For this review, take the finished solid that the model builds, in its own axes (mm). Face numbers are marked on the shaded views. A direction names the side the tool comes from. Coordinates: 2 decimals unless noted, no trailing zeros. Write each loop counter-clockwise with the first axis right and the second up, starting at its lowest first coordinate (ties: lowest second). Pieces come first, ordered by that corner, then holes. Notation, with made-up numbers: (80.5, 37) -> (117.5, 37) arc R23 cw to (117.5, 62) -> close; hole circle Ø3 at (80, 83.5). An arc over 180 degrees is marked (long way). Put each result on its own line as item: value. Start each with the question number.
Item 1: Consider section A-A on x = 0. Give the boundary of the cut face in (y, z).
Item 2: Insertion check: P1, Ø1, axis at y = 7, z = 1, coming from the -X side; P2, Ø1, axis at y = 0, z = 5, coming from the -X side; P3, Ø4, axis at x = 7, z = 1, coming from the +Y side; P4, Ø4, axis at y = -8.5, z = 1.5, coming from the -X side. Each pin has a flat end and moves straight along its axis. Give the tip position at first contact, or say it passes through.
Item 3: The part is to be moulded in two halves that separate along Y. For the marked faces 1, 2 and 3, say which applies: +Y half, -Y half, draft (parallel to the pull), parting line (faces both ways), or undercut.
Item 4: Consider section D-D on x = 3.25. Give the boundary of the cut face in (y, z), and give its area (3 significant figures).
Item 5: Consider section C-C on y = 0. Give the boundary of the cut face in (x, z), and give its area (3 significant figures).
Item 6: For the marked faces 4 and 5, list the 3-axis set-ups (+Z, -Z, +X, -X, +Y, -Y) from which the entire face can be reached by the end or side of a thin tool; tool diameter is ignored.
Item 7: To check wall thickness, follow L1, parallel to Y at x = 0, z = 4.5; L2, parallel to Z at x = 7, y = -9.5; L3, parallel to Y at x = 6.25, z = -2.5. State the ranges of each line that lie inside material, in increasing order.
Item 8: Consider section B-B on z = 7. Give the boundary of the cut face in (x, y).
```python
from build123d import *

# Parameters (mm, degrees)
SKETCH_2_R          = 4.5
EXTRUDE_1_DEPTH     = 9
SKETCH_3_R          = 15
EXTRUDE_2_DEPTH     = 3
CUT_EXTRUDE_1_DEPTH = 10


with BuildPart() as part:
    # Эскиз2 → Бобышка-Вытянуть1 (new body)
    with BuildSketch(Plane.XY):
        Circle(SKETCH_2_R)
    extrude(amount=EXTRUDE_1_DEPTH)

    # Эскиз3 → Бобышка-Вытянуть2 (add)
    with BuildSketch(Plane.XY):
        Circle(SKETCH_3_R)
    extrude(amount=-EXTRUDE_2_DEPTH)

    # Эскиз1 → Вырез-Вытянуть1 (cut)
    with BuildSketch(Plane.XY):
        with BuildLine():
            Line((1.4, 1.697056275), (1.4, -1.697056275))
            ThreePointArc((1.4, -1.697056275), (-2.2, 0), (1.4, 1.697056275))
        make_face()
    extrude(amount=CUT_EXTRUDE_1_DEPTH, mode=Mode.SUBTRACT)


solid = part.part
```
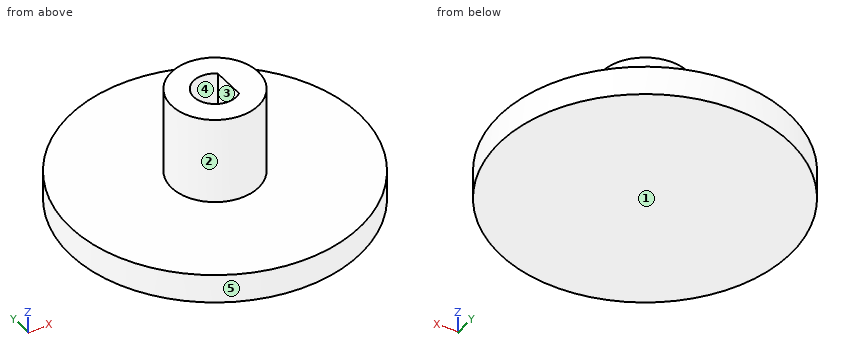
Return value:
1. outline: (-15, -3) -> (15, -3) -> (15, 0) -> (4.5, 0) -> (4.5, 9) -> (2.2, 9) -> (2.2, 0) -> (-2.2, 0) -> (-2.2, 9) -> (-4.5, 9) -> (-4.5, 0) -> (-15, 0) -> close
2. P1: through
2. P2: x = -4.5
2. P3: y = 14.04
2. P4: x = -13.17
3. face 1: draft
3. face 2: parting line
3. face 3: undercut
4. outline: (-14.64, -3) -> (14.64, -3) -> (14.64, 0) -> (3.11, 0) -> (3.11, 9) -> (-3.11, 9) -> (-3.11, 0) -> (-14.64, 0) -> close
4. area: 144 mm^2
5. outline: (-15, -3) -> (15, -3) -> (15, 0) -> (4.5, 0) -> (4.5, 9) -> (1.4, 9) -> (1.4, 0) -> (-2.2, 0) -> (-2.2, 9) -> (-4.5, 9) -> (-4.5, 0) -> (-15, 0) -> close
5. area: 139 mm^2
6. face 4: +Z
6. face 5: +Z, -Z
7. L1: -4.5 to -2.2, 2.2 to 4.5
7. L2: -3 to 0
7. L3: -13.64 to 13.64
8. outline: circle Ø9 at (0, 0); hole (1.4, -1.7) -> (1.4, 1.7) arc R2.2 ccw (long way) to start
